The model under review builds one solid part; all positions refer to its coordinate system, in mm. Face numbers are marked on the shaded views. A direction names the side the tool comes from. Coordinates: 2 decimals unless noted, no trailing zeros. Answer as a JSON object with one key per item and string values.
```python
from build123d import *

# Parameters (mm, degrees)
SKETCH1_W           = 40
SKETCH1_H           = 35
BOSS_EXTRUDE1_DEPTH = 60
SKETCH2_W           = 24.5
SKETCH2_H           = 55
CUT_EXTRUDE1_DEPTH  = 46
BOSS_EXTRUDE2_DEPTH = 3
BOSS_EXTRUDE3_DEPTH = 34
FILLET1_START       = -8
FILLET1_DEPTH       = 3.199770331
FILLET1_START_2     = -17
FILLET1_2_DEPTH     = 34
FILLET2_R           = 16.5
FILLET3_R           = 6
SKETCH5_W           = 20
SKETCH5_H           = 41
CUT_EXTRUDE2_DEPTH  = 68.825143224
SKETCH8_R           = 1.3
SKETCH8_R_2         = 2.5
CUT_EXTRUDE5_DEPTH  = 62.083959026
SKETCH9_R           = 2.15
CUT_EXTRUDE6_DEPTH  = 10


with BuildPart() as part:
    # Sketch1 → Boss-Extrude1 (new body)
    with BuildSketch(Plane(origin=(0, 0, 0), x_dir=(1, 0, 0), z_dir=(0, 1, 0))):
        Rectangle(SKETCH1_W, SKETCH1_H)
    extrude(amount=BOSS_EXTRUDE1_DEPTH)

    # Sketch2 → Cut-Extrude1 (cut)
    with BuildSketch(Plane(origin=(20, 0, 0), x_dir=(0, 0, -1), z_dir=(1, 0, 0))):
        with Locations((-5.25, 32.5)):
            Rectangle(SKETCH2_W, SKETCH2_H)
    extrude(amount=-CUT_EXTRUDE1_DEPTH, mode=Mode.SUBTRACT)

    # Sketch3 → Boss-Extrude2 (add)
    with BuildSketch(Plane(origin=(20, 0, 0), x_dir=(0, 0, -1), z_dir=(1, 0, 0))):
        with BuildLine():
            Line((7, 60), (5.5, 60))
            add(Edge.make_bspline(
                [(5.5, 60), (7.518062239, 25.49671142), (-17.5, 5)],
                knots=[0, 0, 0, 1, 1, 1], degree=2))
            Line((-17.5, 5), (7, 5))
            Line((7, 5), (7, 60))
        make_face()
    boss_extrude2 = extrude(amount=-BOSS_EXTRUDE2_DEPTH)

    # Mirror1: Boss-Extrude2 across plane
    add(boss_extrude2.mirror(Plane(origin=(0, 0, 0), x_dir=(0, 0, 1), z_dir=(1, 0, 0))))

    # Sketch4 → Boss-Extrude3 (add)
    with BuildSketch(Plane.ZY.offset(-17)):
        with BuildLine():
            Line((-7, 60), (-7, 57))
            Line((-7, 57), (-5.625022797, 57))
            add(Edge.make_bspline(
                [(-5.625022797, 57), (-5.588521617, 58.486524947), (-5.499999996, 60.000000071)],
                knots=[0.956135337, 0.956135337, 0.956135337, 1, 1, 1], degree=2))
            Line((-5.499999996, 60.000000071), (-7, 60))
        make_face()
    extrude(amount=BOSS_EXTRUDE3_DEPTH)

    # Fillet1: read off the stored shape, not the designer's step
    # Fillet1 outline → Fillet1 (add)
    with BuildSketch(Plane.XY.offset(FILLET1_START)):
        with BuildLine():
            Line((-17, 57), (-17, 43.5))
            ThreePointArc((-17, 43.5), (-13.045941546, 53.045941546), (-3.5, 57))
            Line((-3.5, 57), (-17, 57))
        make_face()
        with BuildLine():
            Line((17, 57), (3.5, 57))
            ThreePointArc((3.5, 57), (13.045941546, 53.045941546), (17, 43.5))
            Line((17, 43.5), (17, 57))
        make_face()
    extrude(amount=FILLET1_DEPTH)

    # Fillet1 2 outline → Fillet1 2 (cut)
    with BuildSketch(Plane.YZ.offset(FILLET1_START_2)):
        with BuildLine():
            add(Edge.make_bspline(
                [(57, -5.625022797), (49.946623945, -5.798216358), (43.499999985, -4.800229766)],
                knots=[0.043864662, 0.043864662, 0.043864662, 0.251997034, 0.251997034, 0.251997034], degree=2))
            Line((57, -5.625022797), (57, -4.800229669))
            Line((57, -4.800229669), (43.499999985, -4.800229766))
        make_face()
    extrude(amount=FILLET1_2_DEPTH, mode=Mode.SUBTRACT)

    # Fillet2
    # the kernel refuses this fillet: 16.5 mm, written as the material it takes off along each edge
    with BuildSketch(Plane(origin=(20, 60, -58.75), x_dir=(0, -1, 0), z_dir=(0, 0, 1)), Plane(origin=(-20, 60, 35.75), x_dir=(0, -1, 0), z_dir=(0, 0, -1))) as fillet2_piece_1:
        with BuildLine():
            CenterArc((FILLET2_R, -FILLET2_R), FILLET2_R, 90, 90)
            Line((0, -FILLET2_R), (0, 0))
            Line((0, 0), (FILLET2_R, 0))
        make_face()
    extrude(amount=94.5, mode=Mode.SUBTRACT)

    # Fillet3
    # the kernel refuses this fillet: 6 mm, written as the material it takes off along each edge
    with BuildSketch(Plane(origin=(-20, -15, 17.5), x_dir=(0, 0, -1), z_dir=(0, 1, 0))) as fillet3_piece_1:
        with BuildLine():
            CenterArc((FILLET3_R, -FILLET3_R), FILLET3_R, 90, 90)
            Line((0, -FILLET3_R), (0, 0))
            Line((0, 0), (FILLET3_R, 0))
        make_face()
    extrude(amount=35, mode=Mode.SUBTRACT)
    with BuildSketch(Plane(origin=(20, -15, 17.5), x_dir=(0, 0, -1), z_dir=(0, 1, 0))) as fillet3_piece_2:
        with BuildLine():
            CenterArc((FILLET3_R, FILLET3_R), FILLET3_R, 180, 90)
            Line((0, FILLET3_R), (0, 0))
            Line((0, 0), (FILLET3_R, 0))
        make_face()
    extrude(amount=35, mode=Mode.SUBTRACT)

    # Sketch5 → Cut-Extrude2 (cut, through all)
    with BuildSketch(Plane.XY.offset(-7)):
        with Locations((0, 29.5)):
            Rectangle(SKETCH5_W, SKETCH5_H)
    extrude(amount=-CUT_EXTRUDE2_DEPTH, mode=Mode.SUBTRACT)

    # Sketch8 → Cut-Extrude5 (cut, through all)
    with BuildSketch(Plane(origin=(0, 5, 0), x_dir=(1, 0, 0), z_dir=(0, 1, 0))):
        with Locations(Location((-4, 0, 0), (0, 0, 270))):
            Circle(SKETCH8_R)
        with Locations(Location((-8.5, 0, 0), (0, 0, 270))):
            Circle(SKETCH8_R_2)
        with Locations(Location((-13, 0, 0), (0, 0, 270))):
            Circle(SKETCH8_R)
    extrude(amount=-CUT_EXTRUDE5_DEPTH, mode=Mode.SUBTRACT)

    # Sketch9 → Cut-Extrude6 (cut)
    with BuildSketch(Plane(origin=(0, 0, -17.5), x_dir=(-1, 0, 0), z_dir=(0, 0, -1))):
        with Locations((-5, 54.45)):
            Circle(SKETCH9_R)
        with Locations((5, 54.45)):
            Circle(SKETCH9_R)
        with Locations((5, 4.55)):
            Circle(SKETCH9_R)
        with Locations((-5, 4.55)):
            Circle(SKETCH9_R)
    extrude(amount=-CUT_EXTRUDE6_DEPTH, mode=Mode.SUBTRACT)


solid = part.part
```
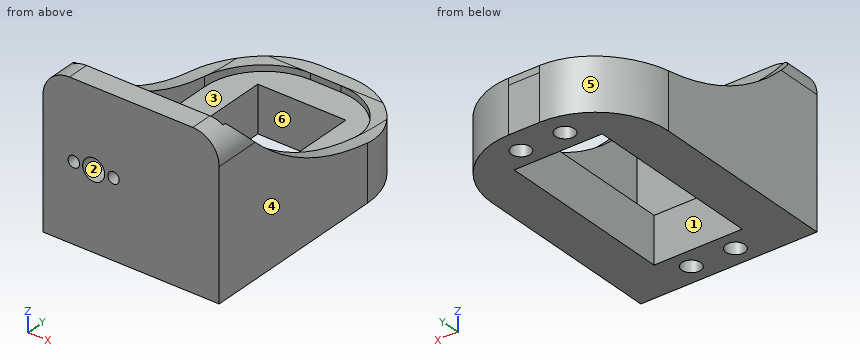
(1) For pin 1 Ø5 at (x, z) = (15.5, -8.5) entering from -Y; pin 2 Ø5 at (x, y) = (-13.5, 36) entering from +Z; pin 3 Ø1.3 at (x, y) = (-6, 54.5) entering from -Z; pin 4 Ø1 at (x, z) = (9, 11) entering from +Y, all flat-tipped, find the tip position at first contact; note any pin that passes through.
Results list:
{"pin 1": "y = 0", "pin 2": "z = -7", "pin 3": "z = -7.5", "pin 4": "y = 5"}
(2) Wall thickness on line 1 along X through (y, z) = (18, -3); line 2 along Y through (x, z) = (0, -13.5); line 3 along X through (y, z) = (3, -8): over which ranges is each line inside the solid? List them lowest first. Write a range as from..to.
Results list:
{"line 1": "-20..-17, 17..20", "line 2": "0..9, 50..60", "line 3": "-20..-6.49, -3.51..3.51, 6.49..20"}
(3) Draft analysis for pull direction X (two halves, no side actions). For the marked faces 4, 5 and 6, state which applies: released by +X, released by -X, zero draft, split by the parting line, or undercut.
Results list:
{"face 4": "released by +X", "face 5": "released by -X", "face 6": "undercut"}
(4) For the marked faces 1, 2 and 3, list the 3-axis set-ups (+Z, -Z, +X, -X, +Y, -Y) from which the entire face can be reached by the end or side of a thin tool; tool diameter is ignored.
Results list:
{"face 1": "+Z, -Z", "face 2": "+Y, -Y", "face 3": "+Z"}
(5) Add section A-A on x = -8.5. Count the separate pieces of the cut face and the enclosed holes in it, and give its area (3 significant figures).
Results list:
{"separate pieces": "3", "enclosed holes": "0", "area": "293 mm²"}
